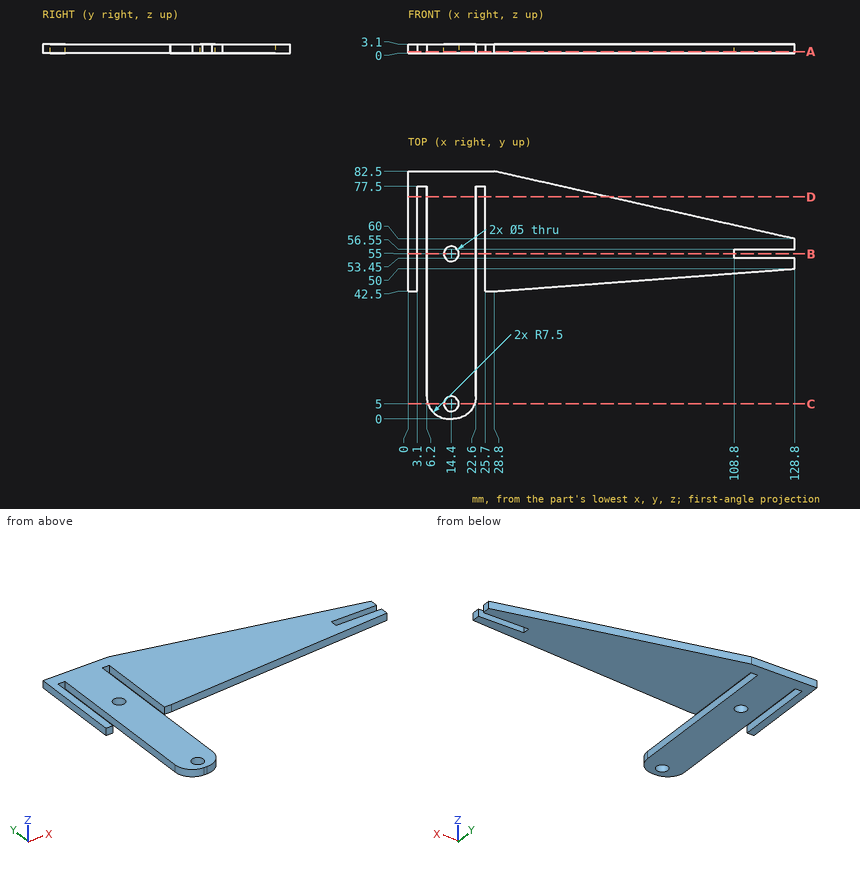
For this review, use the dimensioned drawing (mm, ordinates from the lowest corner) and the shaded views. Give positions to 0.01 mm unless a question says otherwise; leave off trailing zeros. Order: outer loops, then holes, each group sorted by start corner. A loop starts at its lowest first (then second) coordinate and runs counter-clockwise, first axis right, second up.
1. For pin 1 Ø1.6 at (y, z) = (54.5, 1) entering from +X; pin 2 Ø0.9 at (x, z) = (26.5, 2) entering from -Y, all flat-tipped, find the tip position at first contact; note any pin that passes through.
Solution:
pin 1: stops at x = 108.8
pin 2: stops at y = 42.5
2. Add section A-A, the plane z = 0.55. State the section outline as (x, y) points.
Solution:
outline: (0, 42.5) - (3.1, 42.5) - (3.1, 77.5) - (6.2, 77.5) - (6.2, 7.5) arc R7.5 ccw to (13.7, 0) - (15.1, 0) arc R7.5 ccw to (22.6, 7.5) - (22.6, 77.5) - (25.7, 77.5) - (25.7, 42.5) - (28.8, 42.5) - (128.8, 50) - (128.8, 53.45) - (108.8, 53.45) - (108.8, 56.55) - (128.8, 56.55) - (128.8, 60) - (28.8, 82.5) - (0, 82.5) - close; hole circle Ø5 at (14.4, 5); hole circle Ø5 at (14.4, 55)
3. Add section C-C, the plane y = 5. State the section outline as (x, z) points.
Solution:
outline: (6.63, 0) - (11.9, 0) - (11.9, 3.1) - (6.63, 3.1) - close; (16.9, 0) - (22.17, 0) - (22.17, 3.1) - (16.9, 3.1) - close
4. Add section B-B, the plane y = 55. State the section outline as (x, z) points.
Solution:
outline: (0, 0) - (3.1, 0) - (3.1, 3.1) - (0, 3.1) - close; (6.2, 0) - (11.9, 0) - (11.9, 3.1) - (6.2, 3.1) - close; (16.9, 0) - (22.6, 0) - (22.6, 3.1) - (16.9, 3.1) - close; (25.7, 0) - (108.8, 0) - (108.8, 3.1) - (25.7, 3.1) - close
5. Add section D-D, the plane y = 74. State the section outline as (x, z) points.
Solution:
outline: (0, 0) - (3.1, 0) - (3.1, 3.1) - (0, 3.1) - close; (6.2, 0) - (22.6, 0) - (22.6, 3.1) - (6.2, 3.1) - close; (25.7, 0) - (66.58, 0) - (66.58, 3.1) - (25.7, 3.1) - close
6. To check wall thickness, follow L1, parallel to Y at x = 14.4, z = 1.9; L2, parallel to Y at x = 122.5, z = 2.4; L3, parallel to X at y = 18, z = 1.8. State the ranges of each line that lie inside material, in increasing order.
Solution:
L1: y = 0 to 2.5, 7.5 to 52.5, 57.5 to 82.5
L2: y = 49.53 to 53.45, 56.55 to 61.42
L3: x = 6.2 to 22.6
